Input: part model. Units: mm. Frame: model coordinates. Round coordinates to 2 decimals unless told otherwise and drop trailing zeros. Write each loop counter-clockwise with the first axis right and the second up, starting at its lowest first coordinate (ties: lowest second). Pieces come first, ordered by that corner, then holes. Notation, with made-up numbers: M -3.5,86 L 36.5,86 A21 cw 36.5,96 Z; hole C -23.5,39 d6. An arc over 180 degrees is marked long. Write each question's results on one line, items separated by ' | '. Start each with the question number.
Autodesk Inventor part; units mm, degrees
ref_plane "YZ Plane" through (0, 0, 0) normal (1, 0, 0) x (0, 1, 0)
ref_plane "XZ Plane" through (0, 0, 0) normal (0, 1, 0) x (-1, 0, 0)
ref_plane "XY Plane" through (0, 0, 0) normal (0, 0, 1) x (1, 0, 0)
sketch "Sketch1" plane through (0, 0, 0) normal (0, 0, 1) x (1, 0, 0)
  arc A0 (37.1184, 51.5216) -> (-37.1184, 51.5216) centre (0, 0) ccw
  arc A1 (37.8745, 69.7561) -> (-22.5437, 76.1063) centre (0, 0) ccw construction
  arc A2 (52.7268, 71.5758) -> (-52.7268, 71.5758) centre (0, 0) ccw
  circle A3 centre (-22.5437, 76.1063) radius 3.175
  circle A4 centre (37.8745, 69.7561) radius 3.175
  line L0 (37.8745, 69.7561) -> (0, 0) construction
  line L1 (0, 0) -> (-22.5437, 76.1063) construction
  line L2 (0, 79.375) -> (0, 0) construction
  line L3 (-22.5437, 76.1063) -> (0, 79.375) construction
  line L4 (0, 79.375) -> (37.8745, 69.7561) construction
  line L5 (-53.3285, 67.0431) -> (-41.4591, 52.1212)
  line L6 (41.4591, 52.1212) -> (53.3285, 67.0431)
  line L7 (-39.5297, 49.6956) -> (0, 0) construction
  line L8 (0, 0) -> (39.5297, 49.6956) construction
  line L9 (-39.5297, 49.6956) -> (0, 63.5) construction
  line L10 (0, 63.5) -> (39.5297, 49.6956) construction
  arc A5 (-52.7268, 71.5758) -> (-53.3285, 67.0431) centre (-50.8437, 69.0195) ccw
  arc A6 (-41.4591, 52.1212) -> (-37.1184, 51.5216) centre (-38.9743, 54.0977) ccw
  arc A7 (37.1184, 51.5216) -> (41.4591, 52.1212) centre (38.9743, 54.0977) ccw
  arc A8 (53.3285, 67.0431) -> (52.7268, 71.5758) centre (50.8437, 69.0195) ccw
  point P0 (55.3416, 69.5739)
  point P1 (-55.3416, 69.5739)
  dimension "d0" = 79.375
  dimension "d1" = 88.9
  dimension "d2" = 45
  dimension "d5" = 3.175
  dimension "d8" = 6.35
  dimension "d9" = 63.5
  dimension "d10" = 22
  dimension "d11" = 10
extrude "Extrusion1" add sketch "Sketch1" along normal blind 19.05
properties part number "FlyWheel_Weight_Jan21" material "Aluminum-6061"
1. Line query: L1, parallel to X at y = 77, z = 13.25; L2, parallel to X at y = 74, z = 17; L3, parallel to Y at x = -0.5, z = 7. Output: solid intervals per line, ascending. Write a range as from..to.
2. Cut plane B-B on z = 14. Give the number of separate pieces and of enclosed holes in the cut face, and give its area (3 significant figures).
3. Contact query for flat-ended pins moving along their axis: P1, Ø3, axis at x = 2.5, z = 16, coming from the +Y side; P2, Ø5, axis at x = 37.87, y = 69.76, coming from the +Z side; P3, Ø1.5, axis at x = 15, z = 12, coming from the +Y side; P4, Ø8, axis at x = -24.5, z = 12.5, coming from the -Y side. Output: stop coordinate, or through.
4. Cut plane C-C on y = 60.5. Output: boundary loops of the cut face in (x, z).
5. Cut plane A-A on x = 39. Output: boundary loops of the cut face in (y, z), and give its area (3 significant figures).
6. Draft query along X for faces 1 (the face through (-47.48, 59.69, 9.39)), 2 (the face through (47.31, 59.48, 9.39)), 3 (the face through (39.442, 50.957, 9.392)). Return one class per face: +X half, -X half, draft (parallel to the pull), parting line (faces both ways), or undercut.
7. Cut plane D-D on x = -3.5. Output: boundary loops of the cut face in (y, z), and give its area (3 significant figures).
Answers follow:
1) L1: x = -44.43..-25.59, -19.5..44.43 | L2: x = -49.27..-24.92, -20.17..49.27 | L3: y = 63.5..88.9
2) separate pieces: 1 | enclosed holes: 2 | area: 2,530 mm2
3) P1: stops at y = 88.89 | P2: passes through | P3: stops at y = 87.75 | P4: stops at y = 56.75
4) outline: M -48.12,0 L -19.29,0 L -19.29,19.05 L -48.12,19.05 Z; M 19.29,0 L 48.12,0 L 48.12,19.05 L 19.29,19.05 Z
5) outline: M 50.92,0 L 66.79,0 L 66.79,19.05 L 50.92,19.05 Z; M 72.72,0 L 79.89,0 L 79.89,19.05 L 72.72,19.05 Z | area: 439 mm2
6) face 1: -X half | face 2: +X half | face 3: undercut
7) outline: M 63.4,0 L 88.83,0 L 88.83,19.05 L 63.4,19.05 Z | area: 484 mm2
